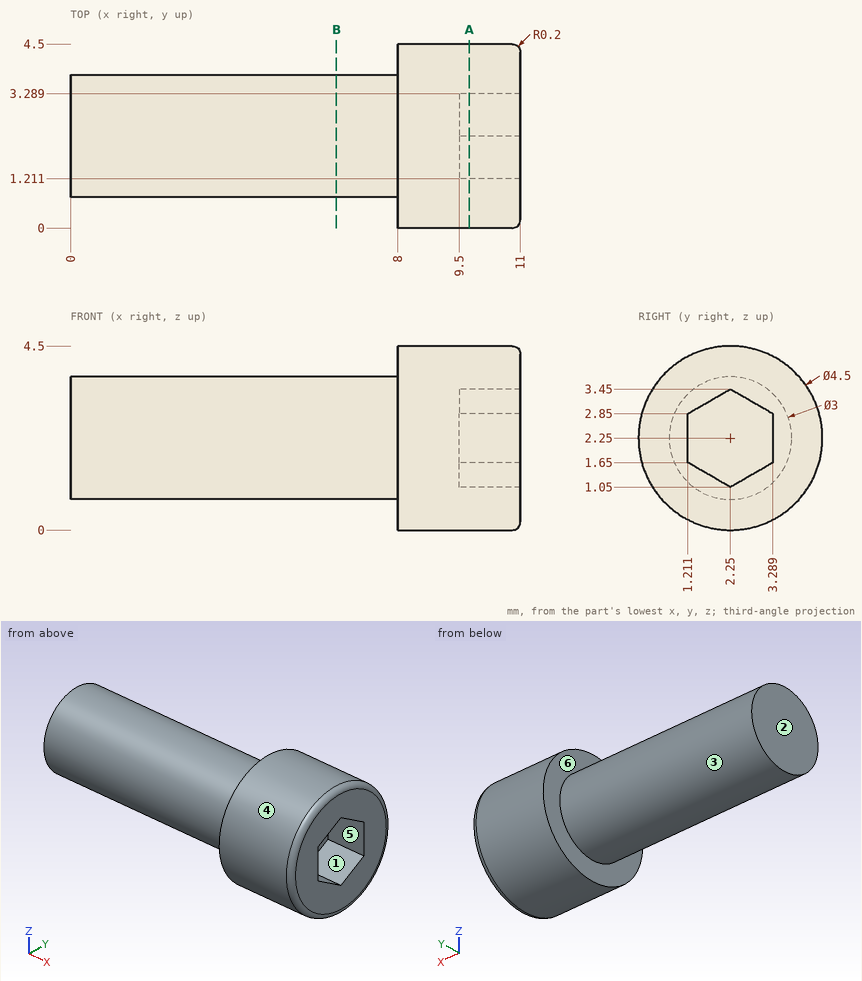
The drawing under review shows one solid part. Ordinate dimensions are in mm from its lowest x, y, z. A direction names the side the tool comes from. Round coordinates to 2 decimals unless told otherwise and drop trailing zeros. Loops run counter-clockwise (first coordinate to the right, second up) from the corner with the lowest first, then second, coordinate; pieces in that order, holes last. Notation, with made-up numbers: (38, 85.25) -> (49, 85.25) arc R4 cw to (49, 90.25) -> close; hole circle Ø6 at (31, 57). An arc over 180 degrees is marked (long way). Answer in a Markdown table with one row per item.
1) Consider section A-A, the plane x = 9.75. Write out the cut boundary in (y, z).
Taken from the geometry:
| item | result |
|---|---|
| outline | circle Ø4.5 at (2.25, 2.25); hole (1.21, 1.65) -> (2.25, 1.05) -> (3.29, 1.65) -> (3.29, 2.85) -> (2.25, 3.45) -> (1.21, 2.85) -> close |
2) For pin 1 Ø1 at (x, z) = (9, 0.5) entering from +Y, flat-tipped, find the tip position at first contact; note if it passes through.
Taken from the geometry:
| item | result |
|---|---|
| pin 1 | stops at y = 4.12 |
3) Consider section B-B, the plane x = 6.5. Write out the cut boundary in (y, z).
Taken from the geometry:
| item | result |
|---|---|
| outline | circle Ø3 at (2.25, 2.25) |
4) Wall thickness on line 1 along X through (y, z) = (1.1, 3.85); line 2 along X through (y, z) = (1.65, 1.45); line 3 along Y through (x, z) = (2.5, 2.15): over which ranges is each line inside the solid? List them lowest first.
Taken from the geometry:
| item | result |
|---|---|
| line 1 | x = 8 to 11 |
| line 2 | x = 0 to 9.5 |
| line 3 | y = 0.75 to 3.75 |
5) Tool access review of the marked faces 4, 5 and 6: name each direction out of +Z, -Z, +X, -X, +Y, -Y from which nothing blocks a thin tool from reaching the whole face with its end or side.
Taken from the geometry:
| item | result |
|---|---|
| face 4 | +X, -X |
| face 5 | +X |
| face 6 | -X |
6) Draft analysis for pull direction Y (two halves, no side actions). For the marked faces 1, 2 and 3, state which applies: pulls with the +Y half, pulls with the -Y half, needs draft (parallel to the pull), parting line crosses it, or undercut.
Taken from the geometry:
| item | result |
|---|---|
| face 1 | undercut |
| face 2 | needs draft |
| face 3 | parting line crosses it |
